Can you work these out from the model? Positions are in its coordinate system, mm. A direction names the side the tool comes from. Give positions to 0.01 mm unless a question says otherwise; leave off trailing zeros.
from build123d import *
from build123d.topology import SkipClean

# Parameters (mm, degrees)
SKETCH1_W           = 25.4
SKETCH1_H           = 25.4
BOSS_EXTRUDE1_DEPTH = 25.4
BOSS_EXTRUDE2_DEPTH = 12.7
SKETCH3_R           = 6.35
BOSS_EXTRUDE3_DEPTH = 6.35
SKETCH4_RX          = 7.099515829
SKETCH4_RY          = 3.549757914
BOSS_EXTRUDE4_DEPTH = 19.05
BOSS_EXTRUDE5_DEPTH = 12.7
SKETCH6_RX          = 16.167018701
SKETCH6_RY          = 10.929819125
BOSS_EXTRUDE6_DEPTH = 1.5875
BOSS_EXTRUDE7_DEPTH = 3.175
BOSS_EXTRUDE8_DEPTH = 3.175


with BuildPart() as part:
    # Sketch1 → Boss-Extrude1 (new body)
    with BuildSketch(Plane(origin=(0, 0, 0), x_dir=(1, 0, 0), z_dir=(0, 1, 0))):
        with Locations((12.7, -12.7)):
            Rectangle(SKETCH1_W, SKETCH1_H)
    extrude(amount=BOSS_EXTRUDE1_DEPTH)

    # Sketch2 → Boss-Extrude2 (add)
    with BuildSketch(Plane(origin=(0, 25.4, 0), x_dir=(1, 0, 0), z_dir=(0, 1, 0))):
        with BuildLine():
            ThreePointArc((6.35, -12.7), (8.209871939, -8.209871939), (12.7, -6.35))
            Line((12.7, -6.35), (19.05, -6.35))
            Line((19.05, -6.35), (19.05, -19.05))
            Line((19.05, -19.05), (6.35, -19.05))
            Line((6.35, -19.05), (6.35, -12.7))
        make_face()
    extrude(amount=BOSS_EXTRUDE2_DEPTH)

    # Sketch3 → Boss-Extrude3 (add)
    with SkipClean():  # keep this step's faces unmerged: merging them makes the solid invalid here
        with BuildSketch(Plane(origin=(0, 38.1, 0), x_dir=(1, 0, 0), z_dir=(0, 1, 0))):
            with Locations(Location((12.7, -12.7, 0), (0, 0, 270))):  # turned: the seam where the file's is
                Circle(SKETCH3_R)
        extrude(amount=BOSS_EXTRUDE3_DEPTH)

    # Sketch4 → Boss-Extrude4 (add)
    with SkipClean():  # keep this step's faces unmerged: merging them makes the solid invalid here
        with BuildSketch(Plane.ZY.offset(-6.35)):
            with Locations(Location((15.875, 31.75), (0, 0, 63.434948823))):
                Ellipse(SKETCH4_RX, SKETCH4_RY)
        extrude(amount=BOSS_EXTRUDE4_DEPTH)

    # Sketch5 → Boss-Extrude5 (add)
    with SkipClean():  # keep this step's faces unmerged: merging them makes the solid invalid here
        with BuildSketch(Plane.ZY):
            Polygon((9.525, 18.199261314), (8.674261314, 16.725738686), (16.725738686, 8.674261314), (19.05, 12.7), (15.875, 18.199261314), align=None)
            Polygon((16.725738686, 8.674261314), (8.674261314, 16.725738686), (6.35, 12.7), (9.525, 7.200738686), (15.875, 7.200738686), align=None)
        extrude(amount=BOSS_EXTRUDE5_DEPTH)

    # Sketch6 → Boss-Extrude6 (add)
    with SkipClean():  # keep this step's faces unmerged: merging them makes the solid invalid here
        with BuildSketch(Plane.ZY.offset(12.7)):
            with Locations(Location((14.2875, 22.650369343), (0, 0, 72.867573148))):
                Ellipse(SKETCH6_RX, SKETCH6_RY)
        extrude(amount=BOSS_EXTRUDE6_DEPTH)

    # Sketch7 → Boss-Extrude7 (add)
    with SkipClean():  # keep this step's faces unmerged: merging them makes the solid invalid here
        with BuildSketch(Plane.ZY.offset(14.2875)):
            Polygon((4.571396825, 23.629289358), (3.732973033, 22.274531466), (3.684255675, 20.682064819), (4.43829853, 19.27858957), (5.793056422, 18.440165778), (7.385523068, 18.391448421), (8.788998317, 19.145491275), (9.627422109, 20.500249167), (9.676139467, 22.092715813), (8.922096612, 23.496191063), (7.56733872, 24.334614855), (5.974872074, 24.383332212), align=None)
            Polygon((9.820093329, 15.591599788), (8.452601667, 14.002128498), (8.609564967, 11.911239943), (10.199036257, 10.54374828), (12.289924812, 10.70071158), (13.657416475, 12.290182871), (13.500453174, 14.381071426), (11.910981884, 15.748563088), align=None)
            Polygon((11.910981884, 27.703541882), (12.440145656, 25.02865315), (15.147636613, 24.705331728), (16.291794276, 27.18039683), (14.291431644, 29.033392611), align=None)
            Polygon((17.003134649, 23.496191063), (13.132029933, 22.83322326), (11.236764719, 19.393318057), (12.744512372, 15.766794232), (16.519908155, 14.684498193), (19.72000204, 16.961420933), (19.935058062, 20.882993187), align=None)
            Polygon((15.755915704, 29.615083354), (23.899741704, 29.243629963), (20.149516777, 36.482116859), align=None)
        extrude(amount=BOSS_EXTRUDE7_DEPTH)

    # Sketch8 → Boss-Extrude8 (add)
    with SkipClean():  # keep this step's faces unmerged: merging them makes the solid invalid here
        with BuildSketch(Plane.XY.offset(25.4)):
            Polygon((16.152157776, 5.413552829), (6.697554447, 9.934608829), (3.837078483, 18.037710904), (8.634948169, 13.986159866), (12.205224218, 19.382989208), (14.110358878, 13.986159866), (11.424856112, 9.926753835), (17.056057389, 9.119429964), (16.152157776, 18.037710904), (19.446911767, 21.939377241), (21.754376792, 16.684574537), (20.669790839, 9.119429964), (20.669790839, 3.810761102), (8.634948169, 2.590986831), (5.267316465, 6.465095533), align=None)
        extrude(amount=BOSS_EXTRUDE8_DEPTH)


solid = part.part
(1) Please list where these lines run through material, in increasing order: probe 1 along X at (y, z) = (25, 16.5); probe 2 along Y at (x, z) = (1.5, 9.5); probe 3 along Y at (x, z) = (8.5, 19).
Returned:
probe 1: x = -14.29 to -12.7, 0 to 25.4
probe 2: y = 0 to 25.4
probe 3: y = 0 to 38.1
(2) Thinking about a two-plate mould opening in Y: for faces 4 (the flat face through (-15.85, 11.48, 12.96)), 5 (the flat face through (17, 12, 28.575)), 6 (the flat face through (-15.85, 19.81, 9.2)), which applies, pulls with the +Y half, pulls with the -Y half, needs draft (parallel to the pull), parting line crosses it, or undercut?
Returned:
face 4: pulls with the -Y half
face 5: needs draft
face 6: undercut
(3) Which directions (+Z, -Z, +X, -X, +Y, -Y) give clear straight access to the entire face, cutting with the end or side of a thin tool? Please do faces 1 (the flat face through (-15.853, 15.055, 12.717)), 2 (the flat face through (6.35, 37, 14)), 3 (the flat face through (13, 32, 19.05)).
Returned:
face 1: -X
face 2: -Z, +Y
face 3: +Z, +X, +Y
(4) Will these pins go through, and if not, where does the flat tip stop? P1, Ø3.5, axis at y = 36.5, z = 15, coming from the -X side; P2, Ø4, axis at x = 15, y = 26.5, coming from the -Z side; P3, Ø1.6, axis at y = 7.5, z = 27.5, coming from the +X side; P4, Ø14, axis at x = 12, y = 33.5, coming from the +Z side.
Returned:
P1: stops at x = -14.29
P2: stops at z = 0
P3: stops at x = 20.67
P4: stops at z = 20.37
